Work out the finished part from the listing and answer in its coordinate system (mm). A direction names the side the tool comes from. Round coordinates to 2 decimals unless told otherwise and drop trailing zeros. Loops run counter-clockwise (first coordinate to the right, second up) from the corner with the lowest first, then second, coordinate; pieces in that order, holes last. Notation, with made-up numbers: (54, -29.75) - (62, -29.75) arc R14 ccw to (62, -14.75) - close; hole circle Ø8 at (10, 68.5). An arc over 180 degrees is marked (long way). Return JSON: item names as keys, results as strings.
from build123d import *

# Parameters (mm, degrees)
BOSS_EXTRUDE1_DEPTH = 58.42


with BuildPart() as part:
    # Sketch1 → Boss-Extrude1 (new body)
    with BuildSketch(Plane(origin=(0, 0, 0), x_dir=(1, 0, 0), z_dir=(0, 1, 0))):
        Polygon((-11, 32.245966686), (0, 32.245966686), (11, 32.245966686), (11, 22.387267321), (28.706556195, 54.137267321), (6.706556195, 63.995966686), align=None)
        Polygon((11, 32.245966686), (0, 32.245966686), (0, 27.316617003), (11, 22.387267321), align=None)
        with BuildLine():
            Line((11, 22.387267321), (0, 27.316617003))
            Line((0, 27.316617003), (0, 24.413342341))
            ThreePointArc((0, 24.413342341), (3.049993619, 23.149993619), (4.313342341, 20.1))
            ThreePointArc((4.313342341, 20.1), (3.049993619, 17.050006381), (0, 15.786657659))
            Line((0, 15.786657659), (0, 4.27242655))
            ThreePointArc((0, 4.27242655), (3.021061785, 3.021061785), (4.27242655, 0))
            ThreePointArc((4.27242655, 0), (3.021061785, -3.021061785), (0, -4.27242655))
            Line((0, -4.27242655), (0, -11.017064321))
            Line((0, -11.017064321), (11, -11.017064321))
            Line((11, -11.017064321), (11, 22.387267321))
        make_face()
        Polygon((0, 27.316617003), (0, 32.245966686), (-11, 32.245966686), align=None)
        with BuildLine():
            Line((0, 24.413342341), (0, 27.316617003))
            Line((0, 27.316617003), (-11, 32.245966686))
            Line((-11, 32.245966686), (-11, -11.017064321))
            Line((-11, -11.017064321), (0, -11.017064321))
            Line((0, -11.017064321), (0, -4.27242655))
            ThreePointArc((0, -4.27242655), (-4.27242655, 0), (0, 4.27242655))
            Line((0, 4.27242655), (0, 15.786657659))
            ThreePointArc((0, 15.786657659), (-4.313342341, 20.1), (0, 24.413342341))
        make_face()
        with BuildLine():
            ThreePointArc((4.313342341, 20.1), (3.049993619, 23.149993619), (0, 24.413342341))
            Line((0, 24.413342341), (0, 15.786657659))
            ThreePointArc((0, 15.786657659), (3.049993619, 17.050006381), (4.313342341, 20.1))
        make_face()
        with BuildLine():
            Line((0, 15.786657659), (0, 24.413342341))
            ThreePointArc((0, 24.413342341), (-4.313342341, 20.1), (0, 15.786657659))
        make_face()
        with BuildLine():
            ThreePointArc((4.27242655, 0), (3.021061785, 3.021061785), (0, 4.27242655))
            Line((0, 4.27242655), (0, -4.27242655))
            ThreePointArc((0, -4.27242655), (3.021061785, -3.021061785), (4.27242655, 0))
        make_face()
        with BuildLine():
            Line((0, -4.27242655), (0, 4.27242655))
            ThreePointArc((0, 4.27242655), (-4.27242655, 0), (0, -4.27242655))
        make_face()
    extrude(amount=BOSS_EXTRUDE1_DEPTH)


solid = part.part
1) Section B-B (x = 19.5) is taken. Give the vertices of the cut face in (y, z).
Verdict:
{"outline": "(0, -58.26) - (58.42, -58.26) - (58.42, -37.63) - (0, -37.63) - close"}
2) Find the intervals of material crossed by L1, parallel to X at y = 42, z = -12.5; L2, parallel to X at y = 7.5, z = -27; L3, parallel to Z at x = 12, y = 11, in increasing order.
Verdict:
{"L1": "x = -11 to 11", "L2": "x = -11 to 13.57", "L3": "z = -61.62 to -24.18"}
3) Section A-A (y = 19.5) is taken. Give the vertices of the cut face in (x, z), and give its area (3 significant figures).
Verdict:
{"outline": "(-11, -32.25) - (6.71, -64) - (28.71, -54.14) - (11, -22.39) - (11, 11.02) - (-11, 11.02) - close", "area": "1,720 mm2"}
4) Flat-ended cylindrical pins translate along their axes: pin 1 (4 mm diameter, centred on x = 11, y = 26.5, fed in from -Z); pin 2 (1.5 mm diameter, centred on x = -0.5, y = 50, fed in from -Z); pin 3 (12 mm diameter, centred on y = 44, z = -40, fed in from -X). Find the tip coordinate at first contact, or state that the pin passes through.
Verdict:
{"pin 1": "stops at z = -62.97", "pin 2": "stops at z = -52.42", "pin 3": "stops at x = -10.02"}
5) Section C-C (z = -49) is taken. Give the vertices of the cut face in (x, y).
Verdict:
{"outline": "(-1.66, 0) - (25.84, 0) - (25.84, 58.42) - (-1.66, 58.42) - close"}
6) A tool of negligible diameter and unlimited length cuts with its end or side. For faces 1 (the flat face through (17.86, 28.8, -59)), 2 (the flat face through (11, 29, -5)), from which of +Z, -Z, +X, -X, +Y, -Y can it reach the whole face along a straight path? Write none if from no direction.
Verdict:
{"face 1": "-Z, +X, +Y, -Y", "face 2": "+Z, +X, +Y, -Y"}
